Could you check a few things on this model? Use its own coordinates, in mm. A direction names the side the tool comes from. Round coordinates to 2 decimals unless told otherwise and drop trailing zeros. Order: outer loops, then holes, each group sorted by start corner. A loop starts at its lowest first (then second) coordinate and runs counter-clockwise, first axis right, second up. Notation, with made-up numbers: (1.5, 26.5) - (59.5, 26.5) arc R10 ccw to (59.5, 34.5) - close; hole circle Ø6 at (25.5, 70.5). An arc over 180 degrees is marked (long way). Use one line per item in the form item = value.
from build123d import *

# Parameters (mm, degrees)
SKETCH1_W                   = 63.5
SKETCH1_H                   = 63.5
BASE_EXTRUDE_DEPTH          = 25.4
SKETCH2_R                   = 28.575
SKETCH2_R_2                 = 25.4
BORE_DEPTH                  = 193.675
SKETCH3_W                   = 63.5
SKETCH3_H                   = 63.5
BOSS_EXTRUDE2_DEPTH         = 38.1
SKETCH4_R                   = 19.05
BOSS_EXTRUDE3_DEPTH         = 22.225
CUT_EXTRUDE1_REACH          = 222.52
SKETCH5_R                   = 12.7
SKETCH6_R                   = 3.96875
TAPPED_BASE_HOLES_MS4_DEPTH = 19.05


with BuildPart() as part:
    # Sketch1 → Base-Extrude (new body)
    with BuildSketch(Plane(origin=(0, 0, 0), x_dir=(0, 0, -1), z_dir=(1, 0, 0))):
        Rectangle(SKETCH1_W, SKETCH1_H)
    extrude(amount=-BASE_EXTRUDE_DEPTH)

    # Sketch2 → BORE (add)
    with BuildSketch(Plane.ZY):
        with Locations(Location((0, 0, 0), (0, 0, 270))):
            Circle(SKETCH2_R)
        with Locations(Location((0, 0, 0), (0, 0, 270))):
            Circle(SKETCH2_R_2, mode=Mode.SUBTRACT)
    extrude(amount=BORE_DEPTH)

    # Sketch3 → Boss-Extrude2 (add)
    with BuildSketch(Plane.ZY.offset(193.675)):
        Rectangle(SKETCH3_W, SKETCH3_H)
    extrude(amount=-BOSS_EXTRUDE2_DEPTH)

    # Sketch4 → Boss-Extrude3 (add)
    with BuildSketch(Plane(origin=(-193.675, 0, 0), x_dir=(0, 0, -1), z_dir=(1, 0, 0))):
        with Locations(Location((0, 0, 0), (0, 0, 90))):
            Circle(SKETCH4_R)
    extrude(amount=-BOSS_EXTRUDE3_DEPTH)

    # Sketch5 → Cut-Extrude1 (cut, up to next)
    with BuildSketch(Plane.ZY.offset(215.9), mode=Mode.PRIVATE) as cut_extrude1_sk1:
        with Locations(Location((0, 0, 0), (0, 0, 270))):
            Circle(SKETCH5_R)
    cut_extrude1_tool1 = extrude(cut_extrude1_sk1.sketch, amount=-CUT_EXTRUDE1_REACH, mode=Mode.PRIVATE) & part.part
    add(cut_extrude1_tool1.solids().sort_by_distance((-215.9, 0, 0))[0], mode=Mode.SUBTRACT)

    # Sketch6 → TAPPED BASE HOLES - MS4 (cut)
    with BuildSketch(Plane(origin=(148.541814714, -31.75, 0.813855987), x_dir=(1, 0, 0), z_dir=(0, -1, 0))):
        with Locations(Location((-161.241814714, 10.298644013, 0), (0, 0, 270))):
            Circle(SKETCH6_R)
        with Locations(Location((-161.241814714, -11.926355987, 0), (0, 0, 270))):
            Circle(SKETCH6_R)
        with Locations(Location((-323.166814714, -11.926355987, 0), (0, 0, 270))):
            Circle(SKETCH6_R)
        with Locations(Location((-323.166814714, 10.298644013, 0), (0, 0, 270))):
            Circle(SKETCH6_R)
    extrude(amount=-TAPPED_BASE_HOLES_MS4_DEPTH, mode=Mode.SUBTRACT)


solid = part.part
Item 1: Imagine slicing it at A-A on z = 0. Please give me the cut outline in (x, y) (3 decimals), plus the area to 3 significant figures.
Found:
outline = (-215.9, -19.05) - (-193.675, -19.05) - (-193.675, -31.75) - (-155.575, -31.75) - (-155.575, -28.575) - (-25.4, -28.575) - (-25.4, -31.75) - (0, -31.75) - (0, 31.75) - (-25.4, 31.75) - (-25.4, 28.575) - (-155.575, 28.575) - (-155.575, 31.75) - (-193.675, 31.75) - (-193.675, 19.05) - (-215.9, 19.05) - (-215.9, 12.7) - (-155.575, 12.7) - (-155.575, 25.4) - (-25.4, 25.4) - (-25.4, -25.4) - (-155.575, -25.4) - (-155.575, -12.7) - (-215.9, -12.7) - close
area = 4,170 mm2
Item 2: Will these pins go through, and if not, where does the flat tip stop? P1, Ø8.5, axis at x = -13.5, z = 12, coming from the -Y side; P2, Ø3, axis at x = -130, y = 3, coming from the -Z side; P3, Ø6.5, axis at x = -12.5, z = -11.5, coming from the -Y side; P4, Ø6, axis at x = -29, y = 14.5, coming from the -Z side.
Found:
P1 = -31.75
P2 = -28.54
P3 = -12.7
P4 = -26.16
Item 3: Imagine slicing it at B-B on x = -12.7. Please give me the cut outline in (y, z), plus the area to 3 significant figures.
Found:
outline = (-31.75, -31.75) - (31.75, -31.75) - (31.75, 31.75) - (-31.75, 31.75) - (-31.75, 15.08) - (-12.7, 15.08) - (-12.7, 7.14) - (-31.75, 7.14) - (-31.75, -7.14) - (-12.7, -7.14) - (-12.7, -15.08) - (-31.75, -15.08) - close
area = 3,730 mm2
Item 4: If we mould it in two halves opening along Z, with no side actions, what happens to faces 4 (the face through (-175, 0, 31.75)), 5 (the face through (-155.575, 12, 5)), 6 (the face through (-175, 31.75, 0))? For each: released by +Z, released by -Z, zero draft, split by the parting line, or undercut.
Found:
face_4 = released by +Z
face_5 = undercut
face_6 = zero draft
Item 5: Imagine slicing it at D-D on z = -21.5. Please give me the cut outline in (x, y) (3 decimals).
Found:
outline = (-193.675, -31.75) - (-155.575, -31.75) - (-155.575, -18.822) - (-25.4, -18.822) - (-25.4, -31.75) - (0, -31.75) - (0, 31.75) - (-25.4, 31.75) - (-25.4, 18.822) - (-155.575, 18.822) - (-155.575, 31.75) - (-193.675, 31.75) - close; hole (-155.575, -13.524) - (-25.4, -13.524) - (-25.4, 13.524) - (-155.575, 13.524) - close
Item 6: Imagine slicing it at C-C on y = 22.5. Please give me the cut outline in (x, z) (3 decimals).
Found:
outline = (-193.675, -31.75) - (-155.575, -31.75) - (-155.575, -17.615) - (-25.4, -17.615) - (-25.4, -31.75) - (0, -31.75) - (0, 31.75) - (-25.4, 31.75) - (-25.4, 17.615) - (-155.575, 17.615) - (-155.575, 31.75) - (-193.675, 31.75) - close; hole (-155.575, -11.786) - (-25.4, -11.786) - (-25.4, 11.786) - (-155.575, 11.786) - close
Item 7: For faces 1 (the face through (-16.221, -22.358, -12.944)), 2 (the face through (-155.575, 0, -29)), 3 (the face through (-13, 0, -31.75)), which set-ups out of +Z, -Z, +X, -X, +Y, -Y let a thin tool reach every point of the face, with its end or its side?
Found:
face_1 = -Y
face_2 = none
face_3 = -Z, +X, -X, +Y, -Y
Item 8: I need wall thicknesses on L1, parallel to X at y = 20.5, z = -14 (3 decimals); L2, parallel to Y at x = -87, z = 0 (3 decimals); L3, parallel to X at y = -13, z = 2 (3 decimals). Which ranges of each line are inside material? Lowest first, please.
Found:
L1 = -193.675 to -155.575, -25.4 to 0
L2 = -28.575 to -25.4, 25.4 to 28.575
L3 = -215.9 to -155.575, -25.4 to 0
